```python
from build123d import *

# Parameters (mm, degrees)
ESQUISSE1_W             = 300
ESQUISSE1_H             = 130
BOSS_EXTRU_1_DEPTH      = 15
ESQUISSE2_R             = 4
ENL_V_MAT_EXTRU_2_DEPTH = 415.976615042
ESQUISSE3_R             = 4
ENL_V_MAT_EXTRU_3_DEPTH = 415.976615042
ESQUISSE5_R             = 4
ENL_V_MAT_EXTRU_4_DEPTH = 415.976615042


with BuildPart() as part:
    # Esquisse1 → Boss.-Extru.1 (new body)
    with BuildSketch(Plane.XY):
        with Locations((-243.802731113, 65)):
            Rectangle(ESQUISSE1_W, ESQUISSE1_H)
    extrude(amount=BOSS_EXTRU_1_DEPTH)

    # Esquisse2 → Enlèv. mat.-Extru.2 (cut, through all)
    with BuildSketch(Plane.XY.offset(15)):
        with Locations((-383.802731113, 120)):
            Circle(ESQUISSE2_R)
    extrude(amount=-ENL_V_MAT_EXTRU_2_DEPTH, mode=Mode.SUBTRACT)

    # Esquisse3 → Enlèv. mat.-Extru.3 (cut, through all)
    with BuildSketch(Plane.XY.offset(15)):
        with Locations((-103.802731113, 10)):
            Circle(ESQUISSE3_R)
    extrude(amount=-ENL_V_MAT_EXTRU_3_DEPTH, mode=Mode.SUBTRACT)

    # Esquisse5 → Enlèv. mat.-Extru.4 (cut, through all)
    with BuildSketch(Plane(origin=(0, 0, 0), x_dir=(-1, 0, 0), z_dir=(0, 0, -1))):
        with Locations((103.802731113, 120)):
            Circle(ESQUISSE5_R)
        with Locations((383.802731113, 10)):
            Circle(ESQUISSE5_R)
    extrude(amount=-ENL_V_MAT_EXTRU_4_DEPTH, mode=Mode.SUBTRACT)


solid = part.part
```
Geometry: final body of the model. Coordinates: model frame, mm. Coordinates: 2 decimals unless noted, no trailing zeros. Order: outer loops, then holes, each group sorted by start corner. A loop starts at its lowest first (then second) coordinate and runs counter-clockwise, first axis right, second up. Notation, with made-up numbers: (36, -19) -> (78, -19) arc R10 cw to (78, -11) -> close; hole circle Ø5 at (-34, 6). An arc over 180 degrees is marked (long way). Use CSV: the item, a comma, the result in double quotes.
1) Section A-A on y = 10. Output: boundary loops of the cut face in (x, z).
Findings:
outline,"(-393.8, 0) -> (-387.8, 0) -> (-387.8, 15) -> (-393.8, 15) -> close; (-379.8, 0) -> (-107.8, 0) -> (-107.8, 15) -> (-379.8, 15) -> close; (-99.8, 0) -> (-93.8, 0) -> (-93.8, 15) -> (-99.8, 15) -> close"
2) Pin query (flat end, axial travel): pin 1 Ø6 at (x, y) = (-261.5, 105) entering from -Z. Return the tip coordinate at first contact, or that it passes through.
Findings:
pin 1,"stops at z = 0"
3) Mould query, pull axis X, two halves, no side actions, for faces 1 (the cylindrical face through (-387.8, 120.18, 7.6)), 2 (the flat face through (-246, 66, 0)), 3 (the flat face through (-93.803, 64, 7)). Classes: +X half, -X half, draft (parallel to the pull), parting line (faces both ways), or undercut.
Findings:
face 1,"undercut"
face 2,"draft"
face 3,"+X half"
